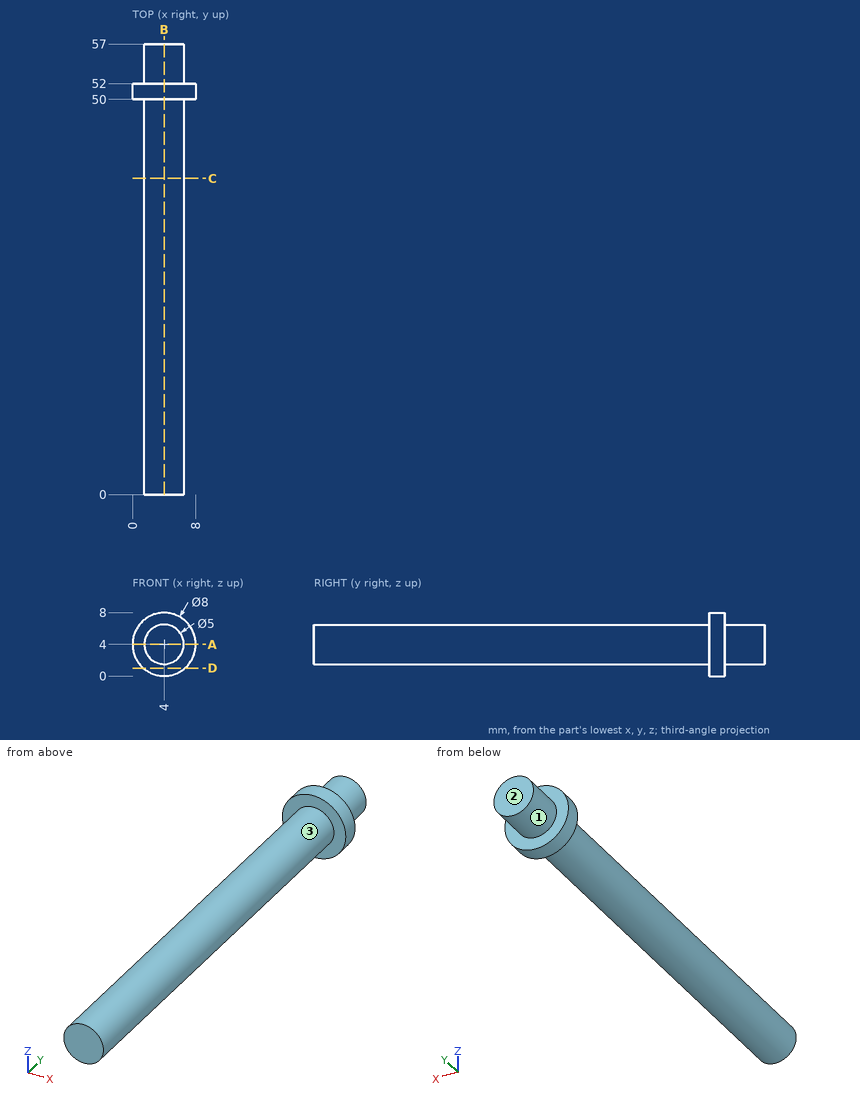
Geometry: see drawing. Coordinates: mm, zero at the bounding-box minimum. A direction names the side the tool comes from. Coordinates: 2 decimals unless noted, no trailing zeros. Write each loop counter-clockwise with the first axis right and the second up, starting at its lowest first coordinate (ties: lowest second). Pieces come first, ordered by that corner, then holes. Notation, with made-up numbers: (83, 80) - (120, 80) arc R31 ccw to (120, 110) - close; hole circle Ø3 at (-34.75, 34). An arc over 180 degrees is marked (long way). Put each result on its own line as item: value. Start each with the question number.
1) Reachability of the marked faces 1, 2 and 3 from +Z, -Z, +X, -X, +Y, -Y: full face, straight path, thin tool, end or side. Return the list, or none.
2) Cut plane D-D (z = 1). Return the cut outline in (x, y).
3) Contact query for flat-ended pins moving along their axis: pin 1 (1 mm diameter, centred on x = 5, y = 33.5, fed in from -Z); pin 2 (2 mm diameter, centred on y = 19.5, z = 5.5, fed in from -X); pin 3 (1 mm diameter, centred on x = 6.5, y = 32.5, fed in from -Z). Output: stop coordinate, or through.
4) Cut plane A-A (z = 4). Return the cut outline in (x, y).
5) Cut plane C-C (y = 40). Return the cut outline in (x, z), plus the area to 3 significant figures.
6) Ray query, L1, parallel to Y at x = 1.75, z = 6; L2, parallel to X at y = 3, z = 2.25; L3, parallel to X at y = 21.5, z = 6.25. Return the intervals inside material, ascending.
7) Cut plane B-B (x = 4). Return the cut outline in (y, z).
Resolved:
1. face 1: +Y
1. face 2: +Z, -Z, +X, -X, +Y
1. face 3: -Y
2. outline: (1.35, 50) - (6.65, 50) - (6.65, 52) - (1.35, 52) - close
3. pin 1: stops at z = 1.55
3. pin 2: stops at x = 1.55
3. pin 3: stops at z = 2.5
4. outline: (0, 50) - (1.5, 50) - (1.5, 0) - (6.5, 0) - (6.5, 50) - (8, 50) - (8, 52) - (6.5, 52) - (6.5, 57) - (1.5, 57) - (1.5, 52) - (0, 52) - close
5. outline: circle Ø5 at (4, 4)
5. area: 19.6 mm2
6. L1: y = 50 to 52
6. L2: x = 2.21 to 5.79
6. L3: x = 2.91 to 5.09
7. outline: (0, 1.5) - (50, 1.5) - (50, 0) - (52, 0) - (52, 1.5) - (57, 1.5) - (57, 6.5) - (52, 6.5) - (52, 8) - (50, 8) - (50, 6.5) - (0, 6.5) - close
